```python
from build123d import *

# Parameters (mm, degrees)
F0_W     = 139.7
F0_H     = 57.15
F1_DEPTH = 3.302
F2_R     = 2.38125
F4_DEPTH = 3.302
F3_R     = 2.38125
F5_DEPTH = 3.302
F6_R     = 2.38125
F7_DEPTH = 3.302
F8_R     = 2.38125
F9_DEPTH = 3.302


with BuildPart() as f1:
    # F0 (on Front) → F1 (new body)
    with BuildSketch(Plane.XZ):
        Rectangle(F0_W, F0_H)
    extrude(amount=F1_DEPTH)

    # F2 (on face) → F4 (cut)
    with BuildSketch(Plane.XZ.offset(3.302)):
        with Locations((-63.5, 22.225)):
            Circle(F2_R)
    extrude(amount=-F4_DEPTH, mode=Mode.SUBTRACT)

    # F3 (on face) → F5 (cut)
    with BuildSketch(Plane.XZ.offset(3.302)):
        with Locations((-63.5, -22.225)):
            Circle(F3_R)
    extrude(amount=-F5_DEPTH, mode=Mode.SUBTRACT)

    # F6 (on face) → F7 (cut)
    with BuildSketch(Plane.XZ.offset(3.302)):
        with Locations((63.5, 22.225)):
            Circle(F6_R)
    extrude(amount=-F7_DEPTH, mode=Mode.SUBTRACT)

    # F8 (on face) → F9 (cut)
    with BuildSketch(Plane.XZ.offset(3.302)):
        with Locations((63.5, -22.225)):
            Circle(F8_R)
    extrude(amount=-F9_DEPTH, mode=Mode.SUBTRACT)


solid = f1.part
```
Build history of the part. All positions in model axes, mm. Coordinates: 2 decimals unless noted, no trailing zeros. Write each loop counter-clockwise with the first axis right and the second up, starting at its lowest first coordinate (ties: lowest second). Pieces come first, ordered by that corner, then holes.
1. Band-saw the part on A-A, the plane x = 63.5. Give the cut face in (y, z) (3 decimals).
Answer block:
outline: (-3.302, -28.575) - (0, -28.575) - (0, -24.606) - (-3.302, -24.606) - close; (-3.302, -19.844) - (0, -19.844) - (0, 19.844) - (-3.302, 19.844) - close; (-3.302, 24.606) - (0, 24.606) - (0, 28.575) - (-3.302, 28.575) - close
2. Drill centre lines: probe 1 along Z at (x, y) = (-63.5, -2.3) (3 decimals); probe 2 along X at (y, z) = (-1.2, 23.5). Where is each one in solid material? Low to high.
Answer block:
probe 1: z = -28.575 to -24.606, -19.844 to 19.844, 24.606 to 28.575
probe 2: x = -69.85 to -65.51, -61.49 to 61.49, 65.51 to 69.85
3. Drop a flat-ended pin along its axis: pin 1 (7.5 mm diameter, centred on x = -63.5, z = -22.225, fed in from -Y). Give the stop position or say it passes through.
Answer block:
pin 1: stops at y = -3.3
4. Pull direction X, two halves, no side cores. Call faces 1 (the cylindrical face through (61.74, -1.67, -20.62)), 2 (the flat face through (-69.85, -2, 0)), 3 (the flat face through (-1, -2, 28.575)): released by +X, released by -X, zero draft, split by the parting line, or undercut.
Answer block:
face 1: undercut
face 2: released by -X
face 3: zero draft
